Design review of the part built by this model. Coordinates are the model's own, in mm. Face numbers are marked on the shaded views. Coordinates: 2 decimals unless noted, no trailing zeros. Write each loop counter-clockwise with the first axis right and the second up, starting at its lowest first coordinate (ties: lowest second). Pieces come first, ordered by that corner, then holes. Notation, with made-up numbers: (-19.5, 42) -> (-9.5, 42) arc R6 ccw to (-9.5, 49) -> close; hole circle Ø9 at (73, -16.75). An arc over 180 degrees is marked (long way). Answer in a Markdown table with one row per item. Add a question column.
Item 1: Draft analysis for pull direction X (two halves, no side actions). For the marked faces 1 and 2, state which applies: released by +X, released by -X, zero draft, split by the parting line, or undercut.
Item 2: Take a section at B-B, the plane x = 0. Write out the cut boundary in (y, z), and give its area (3 significant figures).
Item 3: To check wall thickness, follow line 1 (X direction, y = -0.95, z = 0); line 2 (X direction, y = -0.15, z = -0.5). State the ranges of each line that lie inside material, in increasing order.
Item 4: Take a section at A-A, the plane z = 0. Write out the cut boundary in (x, y).
from build123d import *

# Parameters (mm, degrees)
SKETCH_7_W          = 17
SKETCH_7_H          = 17
EXTRUDE_5_DEPTH     = 1.6
SKETCH_12_R         = 1.05
CUT_EXTRUDE_3_DEPTH = 13.126829759


with BuildPart() as part:
    # 草图7 → 凸台-拉伸5 (new body)
    with BuildSketch(Plane(origin=(0, 0, 0), x_dir=(1, 0, 0), z_dir=(0, 1, 0))):
        Rectangle(SKETCH_7_W, SKETCH_7_H)
    extrude(amount=-EXTRUDE_5_DEPTH)

    # 草图12 → 切除-拉伸3 (cut, through all)
    with BuildSketch(Plane(origin=(0, 0, 0), x_dir=(1, 0, 0), z_dir=(0, 1, 0))):
        with Locations(Location((0, 0, 0), (0, 0, 270))):
            Circle(SKETCH_12_R)
    extrude(amount=-CUT_EXTRUDE_3_DEPTH, mode=Mode.SUBTRACT)


solid = part.part
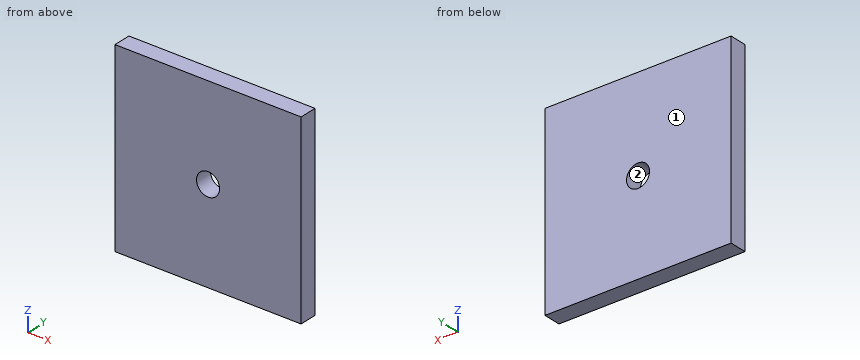
Answers:
| question | item | result |
|---|---|---|
| 1 | face 1 | zero draft |
| 1 | face 2 | undercut |
| 2 | outline | (-1.6, -8.5) -> (0, -8.5) -> (0, -1.05) -> (-1.6, -1.05) -> close; (-1.6, 1.05) -> (0, 1.05) -> (0, 8.5) -> (-1.6, 8.5) -> close |
| 2 | area | 23.8 mm^2 |
| 3 | line 1 | x = -8.5 to -1.05, 1.05 to 8.5 |
| 3 | line 2 | x = -8.5 to -0.92, 0.92 to 8.5 |
| 4 | outline | (-8.5, -1.6) -> (-1.05, -1.6) -> (-1.05, 0) -> (-8.5, 0) -> close; (1.05, -1.6) -> (8.5, -1.6) -> (8.5, 0) -> (1.05, 0) -> close |
